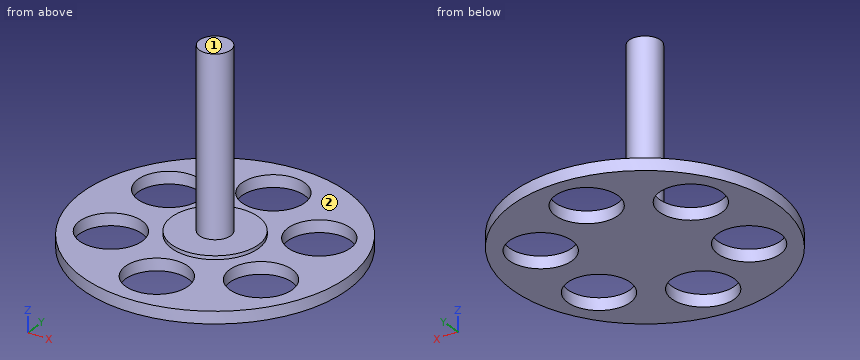
```python
from build123d import *

# Parameters (mm, degrees)
F0_R     = 55
F1_DEPTH = 5
F2_R     = 18
F3_DEPTH = 1.5
F4_R     = 6.5
F5_DEPTH = 73
F6_R     = 13
F7_DEPTH = 5.001


with BuildPart() as f1:
    # F0 (on Top) → F1 (new body)
    with BuildSketch(Plane.XY):
        Circle(F0_R)
    extrude(amount=F1_DEPTH)

    # F2 (on face) → F3 (join)
    with BuildSketch(Plane.XY.offset(5)):
        Circle(F2_R)
    extrude(amount=F3_DEPTH)

    # F4 (on face) → F5 (join)
    with BuildSketch(Plane.XY.offset(6.5)):
        Circle(F4_R)
    extrude(amount=F5_DEPTH)

    # F6 (on face) → F7 (cut, through all)
    with BuildSketch(Plane.XY.offset(5)):
        with Locations((0, 36)):
            Circle(F6_R)
        with Locations((-31.176915, 18)):
            Circle(F6_R)
        with Locations((-31.176915, -18)):
            Circle(F6_R)
        with Locations((0, -36)):
            Circle(F6_R)
        with Locations((31.176915, -18)):
            Circle(F6_R)
        with Locations((31.176915, 18)):
            Circle(F6_R)
    extrude(amount=-F7_DEPTH, mode=Mode.SUBTRACT)


solid = f1.part
```
CAD build for the part. Positions are in the model's coordinates, mm. Face numbers are marked on the shaded views. A direction names the side the tool comes from. Round coordinates to 2 decimals unless told otherwise and drop trailing zeros. Order: outer loops, then holes, each group sorted by start corner. A loop starts at its lowest first (then second) coordinate and runs counter-clockwise, first axis right, second up. Notation, with made-up numbers: (27.5, 54.5) - (41.5, 54.5) arc R12 cw to (41.5, 65.5) - close; hole circle Ø4 at (-40, -30.75). An arc over 180 degrees is marked (long way). Use CSV: the item, a comma, the result in double quotes. Start each with the question number.
1) Saw through at D-D (y = 36). List the corners of the cut face in (x, z), and give its area (3 significant figures).
2) Tool access for the marked faces 1 and 2: list every direction of +Z, -Z, +X, -X, +Y, -Y with a clear straight run to the whole face (end or side of a thin tool).
3) Saw through at C-C (y = 0). List the corners of the cut face in (x, z), and give its area (3 significant figures).
4) Saw through at A-A (x = 0). List the corners of the cut face in (y, z).
5) Wall check: L1, parallel to Y at x = 0, z = 1.1; L2, parallel to Z at x = -21.5, y = -0.5; L3, parallel to Y at x = 0.5, z = 47.5. Give the ranges that are in metal, low to high. Write a range as [from, to].
6) Pin check, flat tips, straight feed: pin 1 Ø10 at (x, y) = (-37.5, 19) entering from -Z; pin 2 Ø8 at (x, y) = (30, 1.5) entering from -Z; pin 3 Ø3 at (y, z) = (5.5, 48) entering from -X; pin 4 Ø3 at (y, z) = (-2.5, 15.5) entering from -X. Stop position of each tip, or through.
7) Saw through at B-B (y = 11.5). List the corners of the cut face in (x, z).
Values follow:
1,outline,"(-41.58, 0) - (-13, 0) - (-13, 5) - (-41.58, 5) - close; (13, 0) - (41.58, 0) - (41.58, 5) - (13, 5) - close"
1,area,"286 mm2"
2,face 1,"+Z, +X, -X, +Y, -Y"
2,face 2,"+Z"
3,outline,"(-55, 0) - (55, 0) - (55, 5) - (18, 5) - (18, 6.5) - (6.5, 6.5) - (6.5, 79.5) - (-6.5, 79.5) - (-6.5, 6.5) - (-18, 6.5) - (-18, 5) - (-55, 5) - close"
3,area,"1,550 mm2"
4,outline,"(-55, 0) - (-49, 0) - (-49, 5) - (-55, 5) - close; (-23, 0) - (23, 0) - (23, 5) - (18, 5) - (18, 6.5) - (6.5, 6.5) - (6.5, 79.5) - (-6.5, 79.5) - (-6.5, 6.5) - (-18, 6.5) - (-18, 5) - (-23, 5) - close; (49, 0) - (55, 0) - (55, 5) - (49, 5) - close"
5,L1,"y = [-55, -49], [-23, 23], [49, 55]"
5,L2,"z = [0, 5]"
5,L3,"y = [-6.48, 6.48]"
6,pin 1,"passes through"
6,pin 2,"stops at z = 0"
6,pin 3,"stops at x = -5.12"
6,pin 4,"stops at x = -6.42"
7,outline,"(-53.78, 0) - (-42.44, 0) - (-42.44, 5) - (-53.78, 5) - close; (-19.92, 0) - (19.92, 0) - (19.92, 5) - (13.85, 5) - (13.85, 6.5) - (-13.85, 6.5) - (-13.85, 5) - (-19.92, 5) - close; (42.44, 0) - (53.78, 0) - (53.78, 5) - (42.44, 5) - close"
